Input: dimensioned drawing with shaded views. Units: mm. Origin: part minimum x, y, z. A direction names the side the tool comes from. Coordinates: 2 decimals unless noted, no trailing zeros. Write each loop counter-clockwise with the first axis right and the second up, starting at its lowest first coordinate (ties: lowest second). Pieces come first, ordered by that corner, then holes. Notation, with made-up numbers: M 60.25,34 L 99.25,34 A17 ccw 99.25,50 Z; hole C 34.5,-27 d7. An arc over 180 degrees is marked long. Use one line per item in the form item = value.
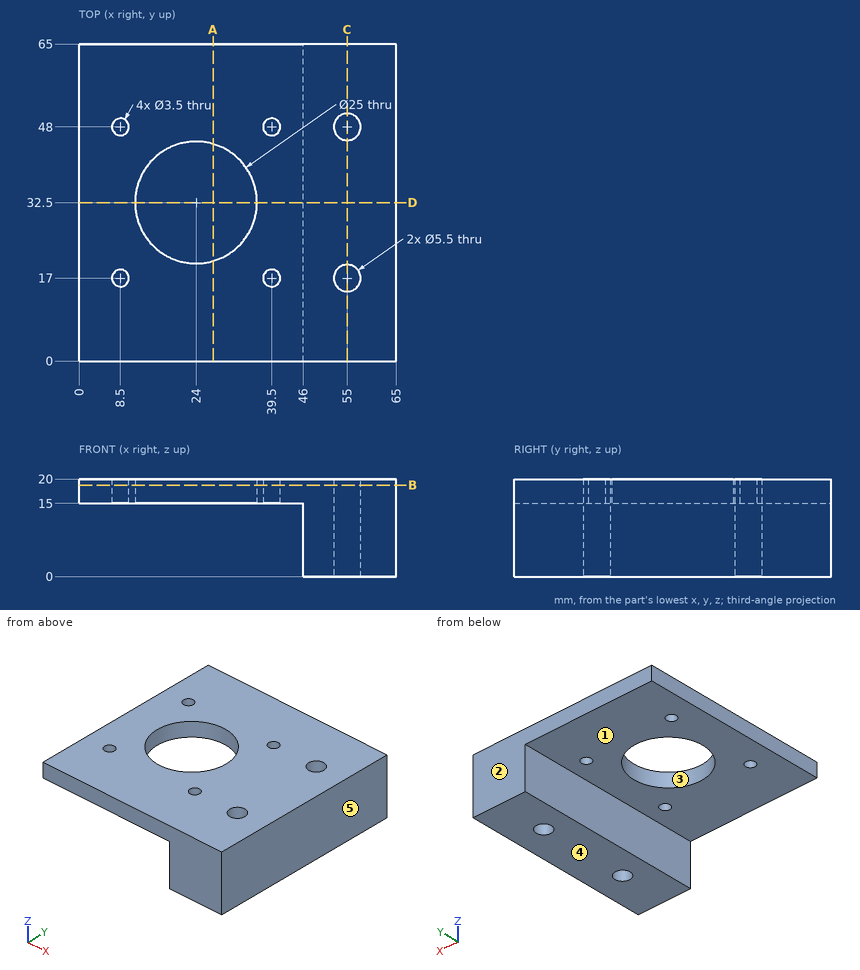
(1) Section query D-D on y = 32.5. Return the cut outline in (x, z), plus the area to 3 significant figures.
Computed:
outline = M 0,15 L 11.5,15 L 11.5,20 L 0,20 Z; M 36.5,15 L 46,15 L 46,0 L 65,0 L 65,20 L 36.5,20 Z
area = 485 mm^2
(2) First-contact query: pin 1 Ø6 at (y, z) = (53, 9.5) entering from -X; pin 2 Ø10 at (x, y) = (16.5, 34.5) entering from -Z; pin 3 Ø4.5 at (x, y) = (55, 17) entering from +Z. Flat tips, straight axial feed; report the tip coordinate or a pass-through.
Computed:
pin_1 = 46
pin_2 = 15
pin_3 = through
(3) Pull-direction query (X, two-part tool) for the marked faces 3, 4 and 5; classes: pulls with the +X half, pulls with the -X half, needs draft (parallel to the pull), parting line crosses it, or undercut.
Computed:
face_3 = undercut
face_4 = needs draft
face_5 = pulls with the +X half
(4) Section query A-A on x = 27.5. Return the cut outline in (y, z).
Computed:
outline = M 0,15 L 20.5,15 L 20.5,20 L 0,20 Z; M 44.5,15 L 65,15 L 65,20 L 44.5,20 Z
(5) Section query B-B on z = 18.75. Return the cut outline in (x, y), plus the area to 3 significant figures.
Computed:
outline = M 0,0 L 65,0 L 65,65 L 0,65 Z; hole C 8.5,17 d3.5; hole C 8.5,48 d3.5; hole C 24,32.5 d25; hole C 39.5,17 d3.5; hole C 39.5,48 d3.5; hole C 55,17 d5.5; hole C 55,48 d5.5
area = 3,650 mm^2
(6) Set-up query: the marked faces 1 and 2. Return all of +Z, -Z, +X, -X, +Y, -Y with unobstructed straight access to the full face (end or side cutting, diameter ignored); none if empty.
Computed:
face_1 = -Z, -X, +Y, -Y
face_2 = +Z, -Z, +X, -X, +Y
(7) Line query: probe 1 along Y at (x, z) = (8.5, 17.5); probe 2 along Y at (x, z) = (55, 6.75); probe 3 along Z at (x, y) = (8, 10). Output: solid intervals per line, ascending.
Computed:
probe_1 = 0 to 15.25, 18.75 to 46.25, 49.75 to 65
probe_2 = 0 to 14.25, 19.75 to 45.25, 50.75 to 65
probe_3 = 15 to 20
(8) Section query C-C on x = 55. Return the cut outline in (y, z).
Computed:
outline = M 0,0 L 14.25,0 L 14.25,20 L 0,20 Z; M 19.75,0 L 45.25,0 L 45.25,20 L 19.75,20 Z; M 50.75,0 L 65,0 L 65,20 L 50.75,20 Z
